Autodesk Inventor part; units mm, degrees
ref_plane "YZ Plane" through (0, 0, 0) normal (1, 0, 0) x (0, 1, 0)
ref_plane "XZ Plane" through (0, 0, 0) normal (0, 1, 0) x (-1, 0, 0)
ref_plane "XY Plane" through (0, 0, 0) normal (0, 0, 1) x (1, 0, 0)
sketch "Sketch1" plane through (0, 0, 0) normal (0, 1, 0) x (-1, 0, 0)
  circle A0 centre (0, 0) radius 6.45
  circle A1 centre (0, 0) radius 5.657
  circle A2 centre (0, 0) radius 2.85
  circle A3 centre (0, 0) radius 1.25
  line L0 (0, 0) -> (-36, 0)
  circle A4 centre (-36, 0) radius 3.5
  line L1 (0, 6.45) -> (-36, 3.5)
  line L2 (0, -6.45) -> (-36, -3.5)
  dimension "d0" = 12.9
  dimension "d1" = 11.314
  dimension "d2" = 5.7
  dimension "d3" = 2.5
  dimension "d4" = 36
  dimension "d5" = 7
extrude "Extrusion1" add sketch "Sketch1" along normal blind 4 contours A0 L2 L1 | A0 L0 A4 L1 | L2 A4 L0 A0 | A4
sketch "Sketch2" plane through (0, 4, 0) normal (0, 1, 0) x (1, 0, 0)
  line L0 (8.4358, -5.7587) -> (8.4358, 5.7587)
  line L1 (8.4358, -5.7587) -> (0, -6.45)
  line L2 (0, -6.45) -> (36, -3.5)
  line L3 (8.4358, 5.7587) -> (0, 6.45)
  line L4 (36, 3.5) -> (0, 6.45)
  arc A0 (0, 6.45) -> (0, -6.45) centre (0, 0) ccw
  arc A1 (0, 6.45) -> (0, -6.45) centre (0, 0) ccw
  circle A2 centre (0, 0) radius 5.657
extrude "Extrusion2" add sketch "Sketch2" along normal blind 1.5
fillet "Fillet1" radius 10 1 edges at (8.4358, 5.5, 0)
sketch "Sketch4" plane through (0, 4, 0) normal (0, 1, 0) x (1, 0, 0)
  circle A0 centre (0, 0) radius 2.9
  dimension "d11" = 5.8
sketch "Sketch5" plane through (0, 4, 0) normal (0, 1, 0) x (1, 0, 0)
  circle A0 centre (0, 0) radius 5.657
extrude "Extrusion3" add sketch "Sketch5" along normal blind 0.5 and the other way blind 2
sketch "Sketch6" plane through (0, 4.5, 0) normal (0, 1, 0) x (1, 0, 0)
  circle A0 centre (0, 0) radius 2.9
  dimension "d17" = 5.8
hole "Hole1" at (0, 4, 0) direction (0, -1, 0) diameter 3 end through all
sketch "Sketch7" plane through (0, 2, 0) normal (0, -1, 0) x (1, 0, 0)
  circle A0 centre (0, 0) radius 2.9
  dimension "d27" = 5.8
hole "Hole2" at (0, 2, 0) direction (0, 1, 0) diameter 5.8 depth 2 tip angle 118
sketch "Sketch9" plane through (0, 4, 0) normal (0, 1, 0) x (1, 0, 0)
  line L0 (8.4358, 5.7587) -> (8.4358, -5.7587)
  arc A0 (36, -3.5) -> (36, 3.5) centre (36, 0) ccw
  circle A1 centre (23.9679, 0) radius 1
  circle A2 centre (34.612, 0) radius 1
  line L1 (0, -6.45) -> (36, -3.5)
  circle A3 centre (29.29, 0) radius 1
  circle A4 centre (13.3238, 0) radius 1
  circle A5 centre (18.6459, 0) radius 1
  point P0 (0, 0)
hole "Hole4" at (13.3238, 4, 0) at (18.6459, 4, 0) at (23.9679, 4, 0) at (29.29, 4, 0) at (34.612, 4, 0) direction (0, -1, 0) diameter 2 end through all
extrude "Extrusion5" cut sketch "Sketch6" against normal blind 0.3
properties part number "servo_arm"
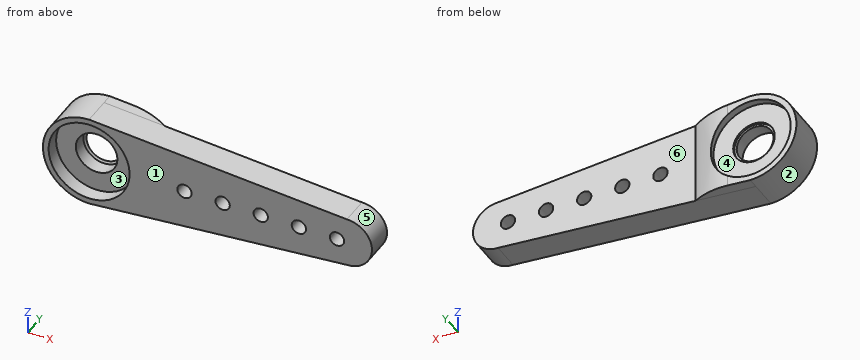
Work out the finished part from the listing and answer in its coordinate system (mm). Face numbers are marked on the shaded views. A direction names the side the tool comes from. Give positions to 0.01 mm unless a question says otherwise; leave off trailing zeros. Order: outer loops, then holes, each group sorted by start corner. A loop starts at its lowest first (then second) coordinate and runs counter-clockwise, first axis right, second up.
1. Section D-D, the plane y = 0.8 is taken. Determine the outline of the cut face in (x, z), and give its area (3 significant figures).
Result sheet:
outline: (0, -6.45) - (36, -3.5) arc R3.5 ccw to (36, 3.5) - (0, 6.45) arc R6.45 ccw to start; hole circle Ø11.31 at (0, 0); hole circle Ø2 at (13.32, 0); hole circle Ø2 at (18.65, 0); hole circle Ø2 at (23.97, 0); hole circle Ø2 at (29.29, 0); hole circle Ø2 at (34.61, 0)
area: 327 mm2
2. Straight lines are drawn through the part: L1, parallel to Z at x = 0, y = 5.3; L2, parallel to Z at x = 0, y = 4.35; L3, parallel to Y at x = 33, z = -0.5. For each, find the intervals that lie inside material, in ascending order.
Result sheet:
L1: z = -6.45 to -5.66, 5.66 to 6.45
L2: z = -6.45 to -2.9, 2.9 to 6.45
L3: y = 0 to 4
3. Each of these flat-tipped pins is pushed along its axis until it touches: P1, Ø5, axis at x = 7, z = 2.5, coming from the +Y side; P2, Ø3.5, axis at x = -2, z = -2, coming from the +Y side; P3, Ø3, axis at y = 2.5, z = -4.5, coming from the +X side. Where does it stop, or does it pass through?
Result sheet:
P1: stops at y = 5.39
P2: stops at y = 4.5
P3: stops at x = 37.8
4. Section A-A, the plane x = 29.29 is taken. Determine the outline of the cut face in (y, z), and give its area (3 significant figures).
Result sheet:
outline: (0, -4.05) - (4, -4.05) - (4, -1) - (0, -1) - close; (0, 1) - (4, 1) - (4, 4.05) - (0, 4.05) - close
area: 24.4 mm2
5. For the marked faces 5 and 6, determine the directions among +Z, -Z, +X, -X, +Y, -Y from which every point of the face is accessible in a straight line to the end or side of a thin tool.
Result sheet:
face 5: +X, +Y, -Y
face 6: +Z, -Z, +X, +Y
6. Section C-C, the plane x = 4 is taken. Determine the outline of the cut face in (y, z), and give its area (3 significant figures).
Result sheet:
outline: (0, -6.12) - (5.47, -6.12) - (5.47, -4) - (4.5, -4) - (4.5, 4) - (5.47, 4) - (5.47, 6.12) - (0, 6.12) - (0, 4) - (2, 4) - (2, -4) - (0, -4) - close
area: 43.2 mm2
7. Section B-B, the plane y = 3 is taken. Determine the outline of the cut face in (x, z).
Result sheet:
outline: (0, -6.45) - (36, -3.5) arc R3.5 ccw to (36, 3.5) - (0, 6.45) arc R6.45 ccw to start; hole circle Ø5.8 at (0, 0); hole circle Ø2 at (13.32, 0); hole circle Ø2 at (18.65, 0); hole circle Ø2 at (23.97, 0); hole circle Ø2 at (29.29, 0); hole circle Ø2 at (34.61, 0)
8. The mould has two halves that part along X. Classify the marked faces 1, 2, 3 and 4: released by +X, released by -X, zero draft, split by the parting line, or undercut.
Result sheet:
face 1: zero draft
face 2: released by -X
face 3: undercut
face 4: undercut
